The model under review builds one solid part; all positions refer to its coordinate system, in mm. Face numbers are marked on the shaded views. A direction names the side the tool comes from. Coordinates: 2 decimals unless noted, no trailing zeros. Write each loop counter-clockwise with the first axis right and the second up, starting at its lowest first coordinate (ties: lowest second). Pieces come first, ordered by that corner, then holes. Notation, with made-up numbers: M 9,24.5 L 61,24.5 A28 cw 61,48.5 Z; hole C 77.5,16.25 d10. An arc over 180 degrees is marked long. Answer as a JSON object with one key per item and string values.
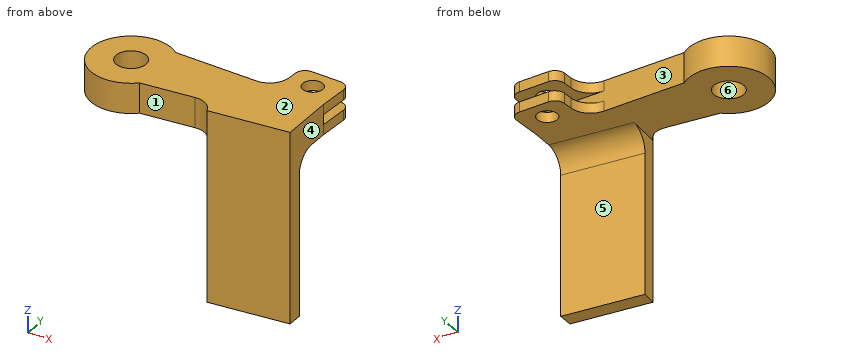
```python
from build123d import *

# Parameters (mm, degrees)
SKETCH1_R                       = 20
SKETCH1_R_2                     = 7.5
BOSS_EXTRUDE1_DEPTH             = 7.5
BOSS_EXTRUDE2_DEPTH             = 7.5
SKETCH4_W                       = 25
SKETCH4_H                       = 5
BOSS_EXTRUDE3_DEPTH             = 20
SKETCH5_R                       = 5
CUT_EXTRUDE1_DEPTH              = 98.765588134
FILLET1_R                       = 5
FILLET2_R                       = 10
BOSS_EXTRUDE4_REACH             = 99.371
BOSS_EXTRUDE4_DIRECTION_2_DEPTH = 80
FILLET3_R                       = 10
FILLET4_R                       = 10


with BuildPart() as part:
    # Sketch1 → Boss-Extrude1 (new, symmetric)
    with BuildSketch(Plane.XY):
        Circle(SKETCH1_R)
        Circle(SKETCH1_R_2, mode=Mode.SUBTRACT)
    extrude(amount=BOSS_EXTRUDE1_DEPTH, both=True)

    # Sketch2 → Boss-Extrude2 (add, symmetric)
    with BuildSketch(Plane.XY):
        with BuildLine():
            Line((13.228756555, 15), (90, 10))
            Line((90, 10), (90, -10))
            Line((90, -10), (13.228756555, -15))
            ThreePointArc((13.228756555, -15), (20, 0), (13.228756555, 15))
        make_face()
    extrude(amount=BOSS_EXTRUDE2_DEPTH, both=True)

    # Sketch4 → Boss-Extrude3 (add)
    with BuildSketch(Plane(origin=(1.028677717, 15.794573482, 0), x_dir=(0.9978858591262095, -0.06499086209573432, 0), z_dir=(0.06499086209573432, 0.9978858591262095, 0))):
        with Locations((76.6598187, 5)):
            Rectangle(SKETCH4_W, SKETCH4_H)
        with Locations((76.6598187, -5)):
            Rectangle(SKETCH4_W, SKETCH4_H)
    extrude(amount=BOSS_EXTRUDE3_DEPTH)

    # Sketch5 → Cut-Extrude1 (cut, through all)
    with BuildSketch(Plane.XY.offset(7.5)):
        with Locations((78.176335382, 20.791244367)):
            Circle(SKETCH5_R)
    extrude(amount=-CUT_EXTRUDE1_DEPTH, mode=Mode.SUBTRACT)

    # Fillet1
    fillet1_edges = [part.edges().sort_by_distance(p)[0] for p in [
        (66.352670764, 31.582488735, -5),
        (91.299817242, 29.957717183, -5),
        (66.352670764, 31.582488735, 5),
        (91.299817242, 29.957717183, 5),
    ]]
    fillet(fillet1_edges, radius=FILLET1_R)

    # Fillet2
    fillet2_edges = [part.edges().sort_by_distance(p)[0] for p in [
        (65.052853522, 11.624771552, -5),
        (65.052853522, 11.624771552, 5),
    ]]
    fillet(fillet2_edges, radius=FILLET2_R)

    # Boss-Extrude4: up to this face of the body (flat: up to its plane)
    boss_extrude4_end = Plane(part.part.faces().sort_by_distance((38.09502008, 2.657537248, 7.5))[0])
    # Sketch6 → Boss-Extrude4 (add, up to the picked face)
    with BuildSketch(Plane(origin=(0, 0, -7.5), x_dir=(-1, 0, 0), z_dir=(0, 0, -1)), mode=Mode.PRIVATE) as boss_extrude4_sk1:
        Polygon((-90, -10), (-90, -17.531812963), (-50, -20.136955084), (-49.511535852, -12.636955084), align=None)
    boss_extrude4_tool1 = split(extrude(boss_extrude4_sk1.sketch, amount=-BOSS_EXTRUDE4_REACH, mode=Mode.PRIVATE), bisect_by=boss_extrude4_end, keep=Keep.BOTH, mode=Mode.PRIVATE)
    add(boss_extrude4_tool1.solids().sort_by(Axis((69.877637, -15.068829, -7.5), (0, 0, 1)))[0])

    # Sketch6 → Boss-Extrude4 direction 2 (add)
    with BuildSketch(Plane(origin=(0, 0, -7.5), x_dir=(-1, 0, 0), z_dir=(0, 0, -1))):
        Polygon((-90, -10), (-90, -17.531812963), (-50, -20.136955084), (-49.511535852, -12.636955084), align=None)
    extrude(amount=BOSS_EXTRUDE4_DIRECTION_2_DEPTH)

    # Fillet3
    # the kernel refuses this fillet: 10 mm, written as the material it adds along each edge
    with BuildSketch(Plane(origin=(49.511535852, -12.636955084, -7.5), x_dir=(0.06499086209573703, -0.9978858591262094, 0), z_dir=(0, 0, 1))) as fillet3_piece_1:
        with BuildLine():
            CenterArc((10, -9.686547154), FILLET3_R, 104.383505331, 75.616494669)
            Line((0, -9.686547154), (0, 0))
            Line((0, 0), (7.51588965, 0))
        make_face()
    extrude(amount=15)

    # Fillet4
    fillet4_edges = [part.edges().sort_by_distance(p)[0] for p in [
        (69.755767926, -11.318477542, -7.5),
    ]]
    fillet(fillet4_edges, radius=FILLET4_R)


solid = part.part
```
(1) For pin 1 Ø1.5 at (x, z) = (9.5, -4) entering from +Y; pin 2 Ø8 at (x, z) = (74.5, -22.5) entering from -Y; pin 3 Ø8 at (x, z) = (75.5, -41) entering from +Y; pin 4 Ø6 at (x, y) = (16.5, 18.5) entering from -Z, all flat-tipped, find the tip position at first contact; note any pin that passes through.
Results list:
{"pin 1": "y = 17.98", "pin 2": "y = -18.8", "pin 3": "y = -10.68", "pin 4": "through"}
(2) Add section D-D on x = 33.5. Give the boundary of the cut face in (y, z).
Results list:
{"outline": "M -13.68,-7.5 L 13.68,-7.5 L 13.68,7.5 L -13.68,7.5 Z"}
(3) Wall thickness on line 1 along Z through (x, y) = (64.5, 14); line 2 along Z through (x, y) = (26, 14); line 3 along Y through (x, z) = (53, -67.5): over which ranges is each line inside the solid? List them lowest first. Write a range as from..to.
Results list:
{"line 1": "-7.5..-2.5, 2.5..7.5", "line 2": "-7.5..7.5", "line 3": "-19.94..-12.41"}
(4) For the marked faces 4, 5 and 6, list the 3-axis set-ups (+Z, -Z, +X, -X, +Y, -Y) from which the entire face can be reached by the end or side of a thin tool; tool diameter is ignored.
Results list:
{"face 4": "+Z, -Z, +X, -Y", "face 5": "-Z, -X, +Y", "face 6": "+Z, -Z"}
(5) Add section C-C on x = 76.5. Count the separate pieces of the cut face and the enclosed holes in it, and give its area (3 significant figures).
Results list:
{"separate pieces": "3", "enclosed holes": "0", "area": "1,170 mm²"}
(6) Draft analysis for pull direction Z (two halves, no side actions). For the marked faces 1, 2 and 3, state which applies: released by +Z, released by -Z, zero draft, split by the parting line, or undercut.
Results list:
{"face 1": "zero draft", "face 2": "released by +Z", "face 3": "undercut"}
(7) Add section A-A on x = 0. Give the boundary of the cut face in (y, z).
Results list:
{"outline": "M -20,-7.5 L -7.5,-7.5 L -7.5,7.5 L -20,7.5 Z; M 7.5,-7.5 L 20,-7.5 L 20,7.5 L 7.5,7.5 Z"}
(8) Add section B-B on z = -53.5. Give the boundary of the cut face in (x, y), and give its area (3 significant figures).
Results list:
{"outline": "M 49.51,-12.64 L 50,-20.14 L 90,-17.53 L 90,-10 Z", "area": "303 mm²"}
